```python
from build123d import *

# Parameters (mm, degrees)
SKETCH_1_R                  = 15
SKETCH_1_R_2                = 12.5
EXTRUDE_1_DEPTH             = 45
SKETCH_2_W                  = 44
SKETCH_2_H                  = 26
SKETCH_2_R                  = 10.5
EXTRUDE_2_DEPTH             = 8
HOLE_WIZARD_M3_1_AT_2_COUNT = 2
HOLE_WIZARD_M3_1_AT_2_PITCH = 35.5
HOLE_WIZARD_M3_1_AT_3_COUNT = 2
HOLE_WIZARD_M3_1_AT_3_PITCH = 25.27968552
SKETCH_6_R                  = 12.5
CUT_EXTRUDE_1_DEPTH         = 43


with BuildPart() as part:
    # 草图1 → 凸台-拉伸1 (new body)
    with BuildSketch(Plane.XY):
        with Locations(Location((0, 0, 0), (0, 0, 180))):
            Circle(SKETCH_1_R)
        with Locations(Location((0, 0, 0), (0, 0, 180))):
            Circle(SKETCH_1_R_2, mode=Mode.SUBTRACT)
    extrude(amount=EXTRUDE_1_DEPTH)

    # 草图2 → 凸台-拉伸2 (add)
    with BuildSketch(Plane.XY.offset(45)):
        Rectangle(SKETCH_2_W, SKETCH_2_H)
        Circle(SKETCH_2_R, mode=Mode.SUBTRACT)
    extrude(amount=-EXTRUDE_2_DEPTH)

    # 草图5 → M3 螺纹孔1 (revolve, cut)
    with BuildSketch(Plane(origin=(-17.75, 13, 41), x_dir=(0, 0, 1), z_dir=(1, 0, 0))):
        Polygon((0, 0), (0, 28), (1.25, 28), (1.25, 0.275), (1.525, 0), align=None)
    hole_wizard_m3_1 = revolve(axis=Axis((-17.75, 19.35, 41), (0, -1, 0)), mode=Mode.SUBTRACT)

    # M3 螺纹孔1 at 2: M3 螺纹孔1 ×2
    with Locations(*[(i * HOLE_WIZARD_M3_1_AT_2_PITCH, 0, 0) for i in range(1, HOLE_WIZARD_M3_1_AT_2_COUNT)]):
        add(hole_wizard_m3_1, mode=Mode.SUBTRACT)

    # M3 螺纹孔1 at 3: M3 螺纹孔1 ×2
    with Locations(*[Vector(0.7021448105364914, 0, -0.7120341740651741) * (i * HOLE_WIZARD_M3_1_AT_3_PITCH) for i in range(1, HOLE_WIZARD_M3_1_AT_3_COUNT)]):
        add(hole_wizard_m3_1, mode=Mode.SUBTRACT)

    # 草图6 → 切除-拉伸1 (cut)
    with BuildSketch(Plane(origin=(0, 0, 0), x_dir=(-1, 0, 0), z_dir=(0, 0, -1))):
        Circle(SKETCH_6_R)
    extrude(amount=-CUT_EXTRUDE_1_DEPTH, mode=Mode.SUBTRACT)


solid = part.part
```
For this review, take the finished solid that the model builds, in its own axes (mm). A direction names the side the tool comes from. Coordinates: 2 decimals unless noted, no trailing zeros. Write each loop counter-clockwise with the first axis right and the second up, starting at its lowest first coordinate (ties: lowest second). Pieces come first, ordered by that corner, then holes.
(1) Tool access review of faces 1 (the face through (-15, -13, 41)), 2 (the face through (-16, 0, 37)), 3 (the face through (15, 13, 41)), 4 (the face through (18, 0, 37)): name each direction out of +Z, -Z, +X, -X, +Y, -Y from which nothing blocks a thin tool from reaching the whole face with its end or side.
(2) Wall thickness on probe 1 along Z at (x, y) = (0, -13.5); probe 2 along Z at (x, y) = (-11.5, 1.5); probe 3 along Z at (x, y) = (-17.75, 0.5): over which ranges is each line inside the solid? List them lowest first.
(3) Add section B-B on x = 0. Give the boundary of the cut face in (y, z) (3 decimals).
(4) Add section D-D on x = -17.75. Give the boundary of the cut face in (y, z) (3 decimals).
(5) The part is to be moulded in two halves that separate along X. For faces 5 (the face through (15, -13, 41)), 6 (the face through (0, 13, 23)), 7 (the face through (-0.05, -13.7, 21.75)), 8 (the face through (22, 0, 41)), say which applies: +X half, -X half, draft (parallel to the pull), parting line (faces both ways), or undercut.
(6) For pin 1 Ø15 at (x, y) = (0, 0) entering from +Z; pin 2 Ø4 at (x, z) = (11.5, 42.5) entering from -Y; pin 3 Ø1 at (x, z) = (-5.5, 39.5) entering from -Y; pin 4 Ø3 at (x, z) = (17.75, 41) entering from +Y (3 decimals), all flat-tipped, find the tip position at first contact; note any pin that passes through.
(7) Add section C-C on y = -4. Give the boundary of the cut face in (x, z).
(8) Add section A-A on z = 41. Give the boundary of the cut face in (x, y) (3 decimals), then the cut area to 3 significant figures.
Answer sheet:
1. face 1: +Z, -Z, -X, -Y
1. face 2: -Z, -X
1. face 3: +Z, -Z, +X, +Y
1. face 4: -Z, +X
2. probe 1: z = 0 to 21.75, 24.25 to 45
2. probe 2: z = 43 to 45
2. probe 3: z = 37 to 39.75, 42.25 to 45
3. outline: (-15, 0) - (-12.5, 0) - (-12.5, 21.75) - (-15, 21.75) - close; (-15, 24.25) - (-12.5, 24.25) - (-12.5, 43) - (-10.5, 43) - (-10.5, 45) - (-15, 45) - close; (10.5, 43) - (12.5, 43) - (12.5, 24.25) - (12.725, 24.25) - (13, 24.525) - (13, 21.475) - (12.725, 21.75) - (12.5, 21.75) - (12.5, 0) - (15, 0) - (15, 45) - (10.5, 45) - close
4. outline: (-13, 37) - (13, 37) - (13, 39.475) - (12.725, 39.75) - (-13, 39.75) - close; (-13, 42.25) - (12.725, 42.25) - (13, 42.525) - (13, 45) - (-13, 45) - close
5. face 5: draft
5. face 6: undercut
5. face 7: undercut
5. face 8: +X half
6. pin 1: passes through
6. pin 2: stops at y = -13
6. pin 3: stops at y = -14.14
6. pin 4: stops at y = 12.975
7. outline: (-22, 37) - (-14.46, 37) - (-14.46, 0) - (-11.84, 0) - (-11.84, 43) - (-9.71, 43) - (-9.71, 45) - (-22, 45) - close; (9.71, 43) - (11.84, 43) - (11.84, 0) - (14.46, 0) - (14.46, 37) - (22, 37) - (22, 45) - (9.71, 45) - close; hole circle Ø2.5 at (-17.75, 41); hole circle Ø2.5 at (17.75, 41)
8. outline: (-22, -13) - (-19, -13) - (-19, 12.725) - (-19.275, 13) - (-22, 13) - close; (-16.5, -13) - (-7.483, -13) arc R15 ccw to (7.483, -13) - (16.5, -13) - (16.5, 12.725) - (16.225, 13) - (7.483, 13) arc R15 ccw to (-7.483, 13) - (-16.225, 13) - (-16.5, 12.725) - close; (19, -13) - (22, -13) - (22, 13) - (19.275, 13) - (19, 12.725) - close; hole circle Ø25 at (0, 0)
8. area: 563 mm2
